Study the drawing (mm; zero at the part's minimum x, y, z) and answer. A direction names the side the tool comes from. Round coordinates to 2 decimals unless told otherwise and drop trailing zeros. Write each loop counter-clockwise with the first axis right and the second up, starting at its lowest first coordinate (ties: lowest second). Pieces come first, ordered by that corner, then holes. Notation, with made-up numbers: (-1, -26.5) - (54, -26.5) arc R13 ccw to (54, -2.5) - close; hole circle Ø4 at (73.5, 50.25). An arc over 180 degrees is marked (long way). Use one line per item in the form item = value. Start each with the question number.
1) The part is cut by section A-A, the plane x = 24. Give the vertices of the cut face in (y, z), plus the area to 4 significant figures.
2) The part is cut by section D-D, the plane y = 17. Give the vertices of the cut face in (x, z), plus the area to 3 significant figures.
3) Consider line 1 along Z through (x, y) = (16.25, 28.5); line 2 along Z through (x, y) = (21, 7.25); line 3 along X through (y, z) = (16, 2.7). Determine where each line is inside the solid, lowest interval first. Write a range as from..to.
4) For the marked faces 1, 2, 3 and 4, determine the directions among +Z, -Z, +X, -X, +Y, -Y from which every point of the face is accessible in a straight line to the end or side of a thin tool.
5) The part is cut by section C-C, the plane y = 9.75. Give the vertices of the cut face in (x, z).
6) Each of these flat-tipped pins is pushed along its axis until it touches: pin 1 (5 mm diameter, centred on x = 24, y = 26, fed in from -Z); pin 2 (0.6 mm diameter, centred on y = 5, z = 1.5, fed in from -X); pin 3 (1.5 mm diameter, centred on x = 13, z = 1.5, fed in from +Y); pin 4 (10 mm diameter, centred on x = 18, y = 17, fed in from -Z). Where does it stop, or does it pass through?
7) The part is cut by section B-B, the plane z = 0.55. Give the vertices of the cut face in (x, y), plus the area to 3 significant figures.
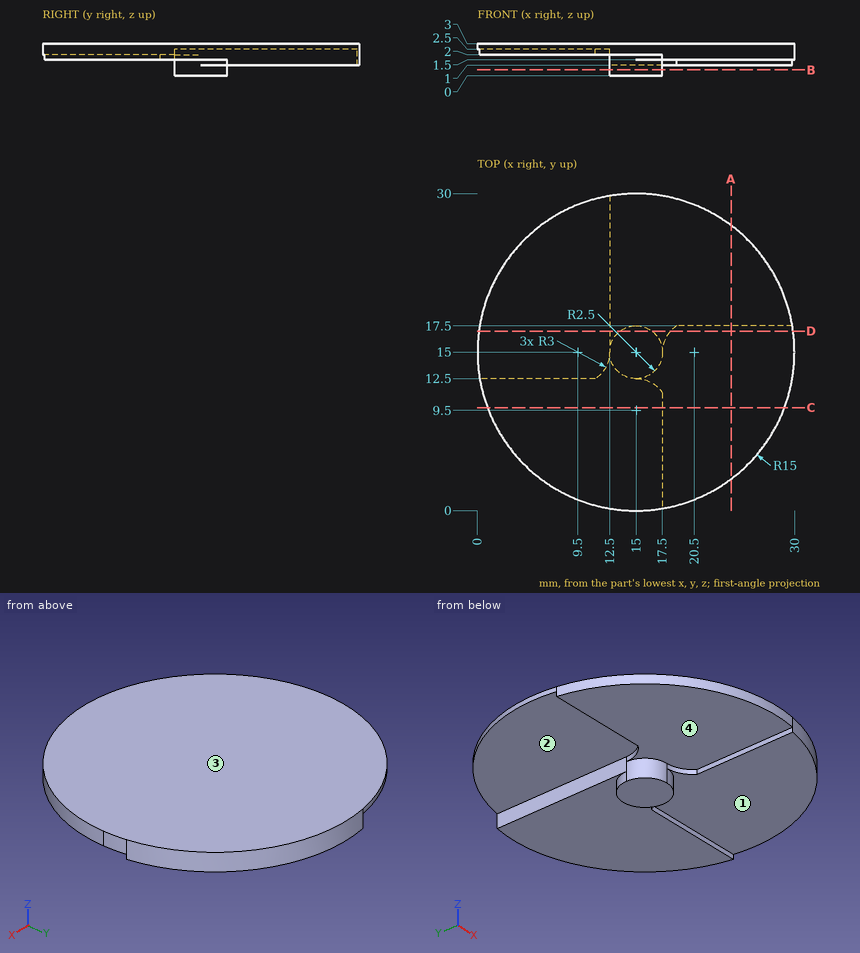
Geometry results:
q1.outline = (3, 1.5) - (17.5, 1.5) - (17.5, 1) - (27, 1) - (27, 3) - (3, 3) - close
q1.area = 40.75 mm2
q2.outline = (0.13, 2.5) - (12.5, 2.5) - (12.5, 1) - (13.5, 1) - (13.5, 0) - (16.5, 0) - (16.5, 1) - (18.26, 1) - (18.26, 1.5) - (29.87, 1.5) - (29.87, 3) - (0.13, 3) - close
q2.area = 38.1 mm2
q3.line_1 = 1..3
q3.line_2 = 1.5..3
q3.line_3 = 0.03..29.97
q4.face_1 = -Z, +X, -Y
q4.face_2 = -Z, -X, +Y
q4.face_3 = +Z, +X, -X, +Y, -Y
q4.face_4 = -Z, -X, -Y
q5.outline = (0.95, 2) - (17.5, 2) - (17.5, 1.5) - (29.05, 1.5) - (29.05, 3) - (0.95, 3) - close
q6.pin_1 = 1
q6.pin_2 = 17.5
q6.pin_3 = 29.95
q6.pin_4 = 0
q7.outline = circle Ø5 at (15, 15)
q7.area = 19.6 mm2
